Study the drawing (mm; zero at the part's minimum x, y, z) and answer. Give positions to 0.01 mm unless a question says otherwise; leave off trailing zeros. Loops run counter-clockwise (first coordinate to the right, second up) from the corner with the lowest first, then second, coordinate; pieces in that order, holes last. Notation, with made-up numbers: M -16.75,85.25 L -11.75,85.25 A23 cw -11.75,124.25 Z; hole C -1.75,72.25 d11. An arc over 180 degrees is marked long. Return JSON: item names as keys, results as strings.
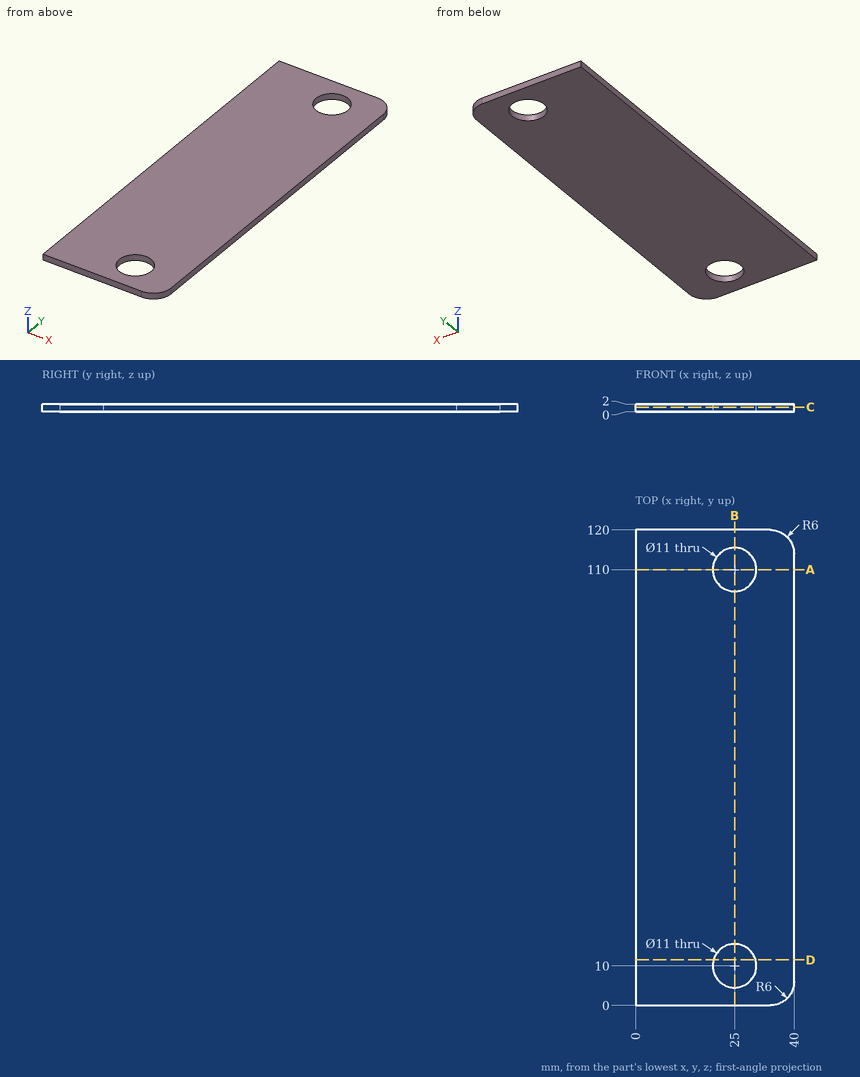
(1) The part is cut by section C-C (z = 1.2). Determine the outline of the cut face in (x, y), and give its area (3 significant figures).
Values follow:
{"outline": "M 0,0 L 34,0 A6 ccw 40,6 L 40,114 A6 ccw 34,120 L 0,120 Z; hole C 25,10 d11; hole C 25,110 d11", "area": "4,590 mm²"}
(2) The part is cut by section A-A (y = 110). Determine the outline of the cut face in (x, z), and give its area (3 significant figures).
Values follow:
{"outline": "M 0,0 L 19.5,0 L 19.5,2 L 0,2 Z; M 30.5,0 L 40,0 L 40,2 L 30.5,2 Z", "area": "58.0 mm²"}
(3) Given pin 1 (1 mm diameter, centred on x = 35.5, z = 1.5, fed in from +Y), flat-ended and moving along its own axis, determine where the tip first touches the part or whether it passes through.
Values follow:
{"pin 1": "y = 119.92"}
(4) The part is cut by section D-D (y = 11.5). Determine the outline of the cut face in (x, z).
Values follow:
{"outline": "M 0,0 L 19.71,0 L 19.71,2 L 0,2 Z; M 30.29,0 L 40,0 L 40,2 L 30.29,2 Z"}
(5) The part is cut by section B-B (x = 25). Determine the outline of the cut face in (y, z).
Values follow:
{"outline": "M 0,0 L 4.5,0 L 4.5,2 L 0,2 Z; M 15.5,0 L 104.5,0 L 104.5,2 L 15.5,2 Z; M 115.5,0 L 120,0 L 120,2 L 115.5,2 Z"}
(6) Straight lines are drawn through the part: line 1 along Y through (x, z) = (25, 1.65); line 2 along Y through (x, z) = (28, 0.6); line 3 along X through (y, z) = (11, 1). For each, find the intervals that lie inside material, in ascending order.
Values follow:
{"line 1": "0 to 4.5, 15.5 to 104.5, 115.5 to 120", "line 2": "0 to 5.39, 14.61 to 105.39, 114.61 to 120", "line 3": "0 to 19.59, 30.41 to 40"}
